The model under review builds one solid part; all positions refer to its coordinate system, in mm. Round coordinates to 2 decimals unless told otherwise and drop trailing zeros. Loops run counter-clockwise (first coordinate to the right, second up) from the corner with the lowest first, then second, coordinate; pieces in that order, holes last. Notation, with made-up numbers: M -21,-39 L 0,-39 A33 cw 0,-9 Z; hole C 47,85 d11. An arc over 180 degrees is marked long. Return JSON: item names as keys, results as strings. Group by question number.
Q1. Consider section A-A (y = 1.5). State the section outline as (x, z) points, and give its area (3 significant figures).
Q2. Clearance check with a flat-ended pin moving along its axis: pin 1 Ø1 at (y, z) = (6, -3) entering from -X. State where the tip first meets the part, or that it passes through.
Q3. To check wall thickness, follow line 1 along Y through (x, z) = (46, -22.5); line 2 along Z through (x, y) = (45.5, 5.5); line 3 along X through (y, z) = (2.75, -20). State the ranges of each line that lie inside material, in increasing order.
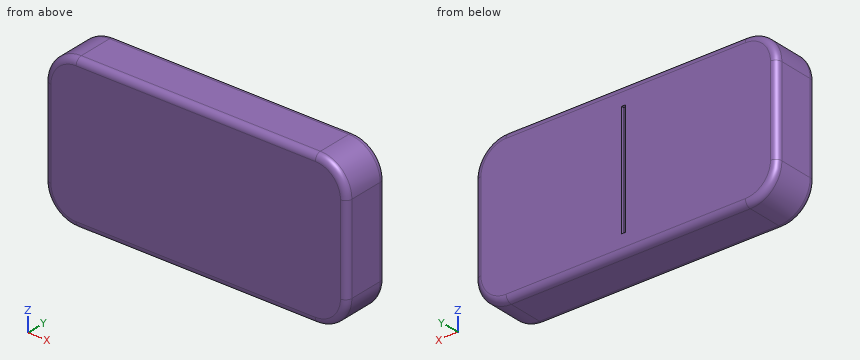
from build123d import *

# Parameters (mm, degrees)
ESQUISSE1_W      = 48
ESQUISSE1_H      = 24
EXTRUSION1_DEPTH = 7.5
CONG_2_R         = 5
CONG_5_R         = 1
CONG_6_R         = 1
ESQUISSE3_W      = 0.662191978
ESQUISSE3_H      = 18
EXTRUSION2_DEPTH = 0.5


with BuildPart() as part:
    # Esquisse1 → Extrusion1 (new body)
    with BuildSketch(Plane(origin=(0, 0, 0), x_dir=(1, 0, 0), z_dir=(0, 1, 0))):
        with Locations((24, 12)):
            Rectangle(ESQUISSE1_W, ESQUISSE1_H)
    extrude(amount=EXTRUSION1_DEPTH)

    # Congé2
    cong_2_edges = [part.edges().sort_by_distance(p)[0] for p in [
        (0, 3.75, -24),
        (48, 3.75, -24),
        (48, 3.75, 0),
        (0, 3.75, 0),
    ]]
    fillet(cong_2_edges, radius=CONG_2_R)

    # Congé5
    cong_5_edges = [part.edges().sort_by_distance(p)[0] for p in [
        (48, 7.5, -12),
        (24, 7.5, 0),
        (0, 7.5, -12),
        (24, 7.5, -24),
        (1.464466094, 7.5, -22.535533906),
        (1.464466094, 7.5, -1.464466094),
        (46.535533906, 7.5, -22.535533906),
        (46.535533906, 7.5, -1.464466094),
    ]]
    fillet(cong_5_edges, radius=CONG_5_R)

    # Congé6
    cong_6_edges = [part.edges().sort_by_distance(p)[0] for p in [
        (48, 0, -12),
        (0, 0, -12),
        (24, 0, -24),
        (24, 0, 0),
        (1.464466094, 0, -22.535533906),
        (1.464466094, 0, -1.464466094),
        (46.535533906, 0, -22.535533906),
        (46.535533906, 0, -1.464466094),
    ]]
    fillet(cong_6_edges, radius=CONG_6_R)

    # Esquisse3 → Extrusion2 (cut)
    with BuildSketch(Plane(origin=(0, 7.5, 0), x_dir=(1, 0, 0), z_dir=(0, 1, 0))):
        with Locations((24.331095989, 12)):
            Rectangle(ESQUISSE3_W, ESQUISSE3_H)
    extrude(amount=-EXTRUSION2_DEPTH, mode=Mode.SUBTRACT)


solid = part.part
Values:
{
 "1": {"outline": "M 0,-19 A5 ccw 5,-24 L 43,-24 A5 ccw 48,-19 L 48,-5 A5 ccw 43,0 L 5,0 A5 ccw 0,-5 Z", "area": "1,130 mm2"},
 "2": {"pin 1": "stops at x = 0.23"},
 "3": {"line 1": "y = 0.21 to 7.29", "line 2": "z = -23.33 to -0.67", "line 3": "x = 0.1 to 47.9"}
}
